The model under review builds one solid part; all positions refer to its coordinate system, in mm. A direction names the side the tool comes from. Coordinates: 2 decimals unless noted, no trailing zeros. Order: outer loops, then holes, each group sorted by start corner. A loop starts at its lowest first (then second) coordinate and runs counter-clockwise, first axis right, second up.
Autodesk Inventor part; units mm, degrees
ref_plane "YZ Plane" through (0, 0, 0) normal (1, 0, 0) x (0, 1, 0)
ref_plane "XZ Plane" through (0, 0, 0) normal (0, 1, 0) x (-1, 0, 0)
ref_plane "XY Plane" through (0, 0, 0) normal (0, 0, 1) x (1, 0, 0)
sketch "スケッチ1" plane through (0, 0, 0) normal (0, 0, 1) x (1, 0, 0)
  line L0 (-31, 46) -> (31, 46)
  line L1 (31, 46) -> (31, -46)
  line L2 (31, -46) -> (-31, -46)
  line L3 (-31, -46) -> (-31, 46)
  point P0 (0, 0)
  dimension "d0" = 92
  dimension "d1" = 46
  dimension "d2" = 62
  dimension "d3" = 31
extrude "押し出し1" add sketch "スケッチ1" along normal blind 1.5
sketch "スケッチ3" plane through (0, 0, 0) normal (0, 0, -1) x (-1, 0, 0)
  circle A0 centre (-7, 26) radius 1.5
  circle A1 centre (15, 26) radius 1.5
  circle A2 centre (-7, -12) radius 1.5
  circle A3 centre (15, -12) radius 1.5
  line L0 (31, 46) -> (-31, 46)
  line L1 (31, -46) -> (31, 46)
  point P0 (0, 0)
  dimension "d10" = 3
  dimension "d11" = 22
  dimension "d12" = 22
  dimension "d15" = 38
  dimension "d16" = 38
  dimension "d35" = 20
  dimension "d36" = 20
  dimension "d44" = 16
  dimension "d45" = 16
hole "穴1" at (-15, -12, 0) at (-15, 26, 0) at (7, 26, 0) at (7, -12, 0) direction (0, 0, 1) diameter 3 end through all
sketch "スケッチ4" plane through (0, 0, 1.5) normal (0, 0, 1) x (1, 0, 0)
  line L0 (-31, -46) -> (-31, 46)
  line L1 (31, -46) -> (-31, -46)
  line L2 (-31, 46) -> (-29.5, 46)
  line L3 (-29.5, 46) -> (-29.5, -46)
  line L4 (-29.5, -46) -> (-31, -46)
  line L5 (-31, -46) -> (-31, 46)
  line L6 (31, 46) -> (29.5, 46)
  line L7 (29.5, 46) -> (29.5, -46)
  line L8 (29.5, -46) -> (31, -46)
  line L9 (31, -46) -> (31, 46)
  point P0 (0, 0)
  dimension "d37" = 59
  dimension "d39" = 1.5
extrude "押し出し3" add sketch "スケッチ4" against normal blind 12.5
sketch "スケッチ6" plane through (31, -46, 0) normal (1, 0, 0) x (0, 0, 1)
  line L0 (1.5, 0) -> (-11, 0)
  line L1 (-11, -92) -> (-5.5, -92)
  line L2 (-5.5, -92) -> (-5.5, 0)
  line L3 (-5.5, 0) -> (-11, 0)
  line L4 (-11, 0) -> (-11, -92)
  point P0 (0, 0)
  point P1 (0, -46)
extrude "押し出し5" cut sketch "スケッチ6" against normal blind 1.5
sketch "スケッチ7" plane through (0, 0, 1.5) normal (0, 0, 1) x (1, 0, 0)
  line L0 (4.5, 13.4115) -> (4.5, 1.4115)
  line L1 (-18.5, 1.4115) -> (-18.5, 13.4115)
  line L2 (-19, 36.9115) -> (8, 36.9115)
  line L3 (-0.3333, 31.9115) -> (-16, 31.9115)
  line L4 (-16, -18.9115) -> (4, -18.9115)
  line L5 (16, -36.9115) -> (-24, -36.9115)
  line L6 (-24, -36.9115) -> (-16, -18.9115)
  line L7 (16, -36.9115) -> (4, -18.9115)
  line L8 (-19, 36.9115) -> (-16, 31.9115)
  line L9 (8, 36.9115) -> (-0.3333, 31.9115)
  arc A0 (-18.5, 1.4115) -> (4.5, 1.4115) centre (-7, 1.4115) ccw
  arc A1 (4.5, 13.4115) -> (-18.5, 13.4115) centre (-7, 13.4115) ccw
  line L10 (31, -46) -> (31, 46)
  line L11 (12, -10.9115) -> (23.5, -28.1615)
  line L12 (23.5, -28.1615) -> (23.5, 26.8385)
  line L13 (23.5, 26.8385) -> (12, 24.0885)
  line L14 (12, -10.9115) -> (12, 24.0885)
  line L15 (29.5, 46) -> (29.5, -46)
  line L16 (-29.5, 46) -> (29.5, 46)
  point P0 (0, 0)
  dimension "d62" = 12
  dimension "d63" = 11.5
  dimension "d64" = 11.5
  dimension "d65" = 23
  dimension "d70" = 5
  dimension "d72" = 18
  dimension "d73" = 27
  dimension "d89" = 40
  dimension "d92" = 20
  dimension "d114" = 35
  dimension "d115" = 55
  dimension "d118" = 11.5
  dimension "d119" = 6
  dimension "d125" = 38
  dimension "d126" = 9.0885
extrude "押し出し7" cut sketch "スケッチ7" against normal blind 1.5
properties material "アセタール樹脂、白"
(1) Draft analysis for pull direction X (two halves, no side actions). For faces 4 (the face through (-31, -1, -5)), 5 (the face through (-15.07, -13.5, 0.76)), 6 (the face through (-2.4, 46, 0.3)), state which applies: released by +X, released by -X, zero draft, split by the parting line, or undercut.
A:
face 4: released by -X
face 5: undercut
face 6: zero draft
(2) We need section A-A, the plane y = 2.5. Write out the cut boundary in (x, z).
A:
outline: (-31, -11) - (-29.5, -11) - (-29.5, 0) - (-18.5, 0) - (-18.5, 1.5) - (-31, 1.5) - close; (4.5, 0) - (12, 0) - (12, 1.5) - (4.5, 1.5) - close; (23.5, 0) - (29.5, 0) - (29.5, -5.5) - (31, -5.5) - (31, 1.5) - (23.5, 1.5) - close
(3) Wall thickness on probe 1 along Y at (x, z) = (-4, 0.5); probe 2 along X at (y, z) = (-12, 1.2); probe 3 along Y at (x, z) = (7, 0.5): over which ranges is each line inside the solid? List them lowest first.
A:
probe 1: y = -46 to -36.91, -18.91 to -9.69, 24.51 to 31.91, 36.91 to 46
probe 2: x = -31 to -16.5, -13.5 to 5.5, 8.5 to 12.73, 23.5 to 31
probe 3: y = -46 to -36.91, -23.41 to -13.5, -10.5 to 24.5, 27.5 to 36.31, 36.91 to 46
(4) We need section D-D, the plane x = -7. Write out the cut boundary in (y, z), and give its area (3 significant figures).
A:
outline: (-46, 0) - (-36.91, 0) - (-36.91, 1.5) - (-46, 1.5) - close; (-18.91, 0) - (-10.09, 0) - (-10.09, 1.5) - (-18.91, 1.5) - close; (24.91, 0) - (31.91, 0) - (31.91, 1.5) - (24.91, 1.5) - close; (36.91, 0) - (46, 0) - (46, 1.5) - (36.91, 1.5) - close
area: 51.0 mm2
(5) Machinability: for faces 1 (the face through (31, 1, -2)), 2 (the face through (17.83, 25.483, 0.76)), 3 (the face through (29.5, 1, -3)), which of the approach directions +Z, -Z, +X, -X, +Y, -Y give a long, thin tool a straight path to every point of the face, cutting with its end or side? Answer none if there is none.
A:
face 1: +Z, -Z, +X, +Y, -Y
face 2: +Z, -Z
face 3: -Z, +Y, -Y
(6) For pin 1 Ø4 at (x, y) = (7, 26) entering from -Z, flat-tipped, find the tip position at first contact; note if it passes through.
A:
pin 1: stops at z = 0
(7) We need section B-B, the plane z = -1.75. Write out the cut boundary in (x, y).
A:
outline: (-31, -46) - (-29.5, -46) - (-29.5, 46) - (-31, 46) - close; (29.5, -46) - (31, -46) - (31, 46) - (29.5, 46) - close
(8) We need section C-C, the plane x = -15. Write out the cut boundary in (y, z), and give its area (3 significant figures).
A:
outline: (-46, 0) - (-36.91, 0) - (-36.91, 1.5) - (-46, 1.5) - close; (-18.91, 0) - (-13.5, 0) - (-13.5, 1.5) - (-18.91, 1.5) - close; (-10.5, 0) - (-6.85, 0) - (-6.85, 1.5) - (-10.5, 1.5) - close; (21.67, 0) - (24.5, 0) - (24.5, 1.5) - (21.67, 1.5) - close; (27.5, 0) - (31.91, 0) - (31.91, 1.5) - (27.5, 1.5) - close; (36.91, 0) - (46, 0) - (46, 1.5) - (36.91, 1.5) - close
area: 51.7 mm2
